```python
from build123d import *

# Parameters (mm, degrees)
CUT_EXTRUDE1_DEPTH = 2


with BuildPart() as part:
    # Sketch1 → Revolve1 (revolve)
    with BuildSketch(Plane(origin=(0, 0, 0), x_dir=(0, 0, -1), z_dir=(1, 0, 0)), mode=Mode.PRIVATE) as revolve1_sk:
        with BuildLine():
            Line((0, 3), (0, -8))
            Line((0, -8), (1.3, -8))
            Line((1.3, -8), (1.5, -7.8))
            Line((1.5, -7.8), (1.5, -0.2))
            ThreePointArc((1.5, -0.2), (1.558578644, -0.058578644), (1.7, 0))
            Line((1.7, 0), (2.7, 0))
            Line((2.7, 0), (2.7, 2.8))
            ThreePointArc((2.7, 2.8), (2.641421356, 2.941421356), (2.5, 3))
            Line((2.5, 3), (0, 3))
        make_face()
    revolve(revolve1_sk.sketch.rotate(Axis((0, 11.82745098, 0), (0, -1, 0)), 180), axis=Axis((0, 11.82745098, 0), (0, -1, 0)))

    # Sketch2 → Cut-Extrude1 (cut)
    with BuildSketch(Plane(origin=(0, 3, 0), x_dir=(1, 0, 0), z_dir=(0, 1, 0))):
        Polygon((0.721687836, 1.25), (-0.721687836, 1.25), (-1.443375673, 0), (-0.721687836, -1.25), (0.721687836, -1.25), (1.443375673, 0), align=None)
    extrude(amount=-CUT_EXTRUDE1_DEPTH, mode=Mode.SUBTRACT)


solid = part.part
```
The listing builds one solid part. Answer for the finished solid, in the listing's coordinates (mm). A direction names the side the tool comes from. Give positions to 0.01 mm unless a question says otherwise; leave off trailing zeros. Loops run counter-clockwise (first coordinate to the right, second up) from the corner with the lowest first, then second, coordinate; pieces in that order, holes last. Notation, with made-up numbers: (42.5, 25.25) - (66.5, 25.25) arc R15 ccw to (66.5, 33.25) - close; hole circle Ø9 at (81.25, 67.5). An arc over 180 degrees is marked (long way). Answer as CSV lines item,"result". Start each with the question number.
Item 1: A cutting plane is placed at B-B on y = -2.5. Determine the outline of the cut face in (x, z), then the cut area to 3 significant figures.
Item 2: A cutting plane is placed at A-A on y = 2. Determine the outline of the cut face in (x, z), then the cut area to 3 significant figures.
Item 3: For faces 1 (the face through (0, 2, -1.25)), 2 (the face through (2, 0, 0)), 3 (the face through (1.643, 1.42, -2.143)), determine the directions among +Z, -Z, +X, -X, +Y, -Y from which every point of the face is accessible in a straight line to the end or side of a thin tool.
Item 4: Find the intervals of material crossed by line 1 (Z direction, x = -0.1, y = 2.25); line 2 (Y direction, x = 2.4, z = 0.35); line 3 (Z direction, x = 0.1, y = -7.5), in increasing order. Write a range as from..to.
Item 5: The mould has two halves that part along Z. Classify faces 4 (the face through (0, 2, 1.25)), 5 (the face through (-0.45, -3.95, 1.43)), 6 (the face through (1.1, 3, 1.1)): +Z half, -Z half, draft (parallel to the pull), parting line (faces both ways), or undercut.
Item 6: Each of these flat-tipped pins is pushed along its axis until it touches: pin 1 (2 mm diameter, centred on x = 1.5, y = -4, fed in from -Z); pin 2 (3 mm diameter, centred on x = -0.5, y = -3, fed in from +Z); pin 3 (1 mm diameter, centred on x = -2, z = 1, fed in from -Y). Where does it stop, or does it pass through?
Found:
1,outline,"circle Ø3 at (0, 0)"
1,area,"7.07 mm^2"
2,outline,"circle Ø5.4 at (0, 0); hole (-1.44, 0) - (-0.72, -1.25) - (0.72, -1.25) - (1.44, 0) - (0.72, 1.25) - (-0.72, 1.25) - close"
2,area,"17.5 mm^2"
3,face 1,"+Y"
3,face 2,"-Y"
3,face 3,"+Y, -Y"
4,line 1,"z = -2.7..-1.25, 1.25..2.7"
4,line 2,"y = 0..3"
4,line 3,"z = -1.5..1.5"
5,face 4,"undercut"
5,face 5,"parting line"
5,face 6,"draft"
6,pin 1,"stops at z = -1.41"
6,pin 2,"stops at z = 1.5"
6,pin 3,"stops at y = 0"
